The model under review builds one solid part; all positions refer to its coordinate system, in mm. A direction names the side the tool comes from. Round coordinates to 2 decimals unless told otherwise and drop trailing zeros. Write each loop counter-clockwise with the first axis right and the second up, starting at its lowest first coordinate (ties: lowest second). Pieces come first, ordered by that corner, then holes. Notation, with made-up numbers: (76, 53.5) - (125, 53.5) arc R14 ccw to (125, 73.5) - close; hole circle Ø6 at (-19, -15). An arc over 180 degrees is marked (long way). One line per question, with ' | ' between items. Start each with the question number.
```python
from build123d import *

# Parameters (mm, degrees)
SKETCH_1_W          = 23
SKETCH_1_H          = 32
EXTRUDE_1_DEPTH     = 6.5
SKETCH_3_W          = 18.5
SKETCH_3_H          = 32
CUT_EXTRUDE_1_DEPTH = 3.8
SKETCH_4_W          = 23.00306398
SKETCH_4_H          = 3
CUT_EXTRUDE_2_DEPTH = 2
SKETCH_5_R          = 0.6
CUT_EXTRUDE_3_DEPTH = 7.5
SKETCH_6_W          = 5
SKETCH_6_H          = 7
EXTRUDE_2_DEPTH     = 8.5
FILLET_1_R          = 1
SKETCH_7_R          = 0.5
CUT_EXTRUDE_4_DEPTH = 24
FILLET_2_R          = 2
FILLET_3_R          = 1
SKETCH_8_W          = 4
SKETCH_8_H          = 5
CUT_EXTRUDE_5_DEPTH = 16
SKETCH_9_R          = 1
CUT_EXTRUDE_6_DEPTH = 3
SKETCH_10_W         = 1
SKETCH_10_H         = 28
CUT_EXTRUDE_7_DEPTH = 7.5


with BuildPart() as part:
    # 草图1 → 凸台-拉伸1 (new body)
    with BuildSketch(Plane(origin=(0, 0, 0), x_dir=(1, 0, 0), z_dir=(0, 1, 0))):
        Rectangle(SKETCH_1_W, SKETCH_1_H)
    extrude(amount=EXTRUDE_1_DEPTH)

    # 草图3 → 切除-拉伸1 (cut)
    with BuildSketch(Plane.XZ):
        Rectangle(SKETCH_3_W, SKETCH_3_H)
    extrude(amount=-CUT_EXTRUDE_1_DEPTH, mode=Mode.SUBTRACT)

    # 草图4 → 切除-拉伸2 (cut)
    with BuildSketch(Plane.XZ):
        with Locations((0.00153199, 3.5)):
            Rectangle(SKETCH_4_W, SKETCH_4_H)
        with Locations((0.00153199, -3.5)):
            Rectangle(SKETCH_4_W, SKETCH_4_H)
    extrude(amount=-CUT_EXTRUDE_2_DEPTH, mode=Mode.SUBTRACT)

    # 草图5 → 切除-拉伸3 (cut, through all)
    with BuildSketch(Plane.XZ):
        with Locations((-10.375, -8)):
            Circle(SKETCH_5_R)
        with Locations((10.375, -8)):
            Circle(SKETCH_5_R)
        with Locations((10.375, 8)):
            Circle(SKETCH_5_R)
        with Locations((-10.375, 8)):
            Circle(SKETCH_5_R)
    extrude(amount=-CUT_EXTRUDE_3_DEPTH, mode=Mode.SUBTRACT)

    # 草图6 → 凸台-拉伸2 (add)
    with BuildSketch(Plane(origin=(0, 6.5, 0), x_dir=(1, 0, 0), z_dir=(0, 1, 0))):
        with Locations((9, 0)):
            Rectangle(SKETCH_6_W, SKETCH_6_H)
    extrude(amount=EXTRUDE_2_DEPTH)

    # 圆角1
    fillet_1_edges = [part.edges().sort_by_distance(p)[0] for p in [
        (10.375, 2, 5),
        (-10.375, 2, 5),
        (10.375, 2, 2),
        (-10.375, 2, 2),
        (10.375, 2, -5),
        (-10.375, 2, -5),
        (10.375, 2, -2),
        (-10.375, 2, -2),
    ]]
    fillet(fillet_1_edges, radius=FILLET_1_R)

    # 草图7 → 切除-拉伸4 (cut, through all)
    with BuildSketch(Plane(origin=(11.5, 0, 0), x_dir=(0, 0, -1), z_dir=(1, 0, 0))):
        with Locations((-2, 10.75)):
            Circle(SKETCH_7_R)
        with Locations((2, 10.75)):
            Circle(SKETCH_7_R)
    extrude(amount=-CUT_EXTRUDE_4_DEPTH, mode=Mode.SUBTRACT)

    # 圆角2
    fillet_2_edges = [part.edges().sort_by_distance(p)[0] for p in [
        (9, 15, 3.5),
        (9, 15, -3.5),
    ]]
    fillet(fillet_2_edges, radius=FILLET_2_R)

    # 圆角3
    fillet_3_edges = [part.edges().sort_by_distance(p)[0] for p in [
        (6.5, 6.5, 0),
        (9, 6.5, 3.5),
        (9, 6.5, -3.5),
    ]]
    fillet(fillet_3_edges, radius=FILLET_3_R)

    # 草图8 → 切除-拉伸5 (cut, through all)
    with BuildSketch(Plane.XZ):
        with Locations((9.5, 13.5)):
            Rectangle(SKETCH_8_W, SKETCH_8_H)
        with Locations((9.5, -13.5)):
            Rectangle(SKETCH_8_W, SKETCH_8_H)
    extrude(amount=-CUT_EXTRUDE_5_DEPTH, mode=Mode.SUBTRACT)

    # 草图9 → 切除-拉伸6 (cut)
    with BuildSketch(Plane(origin=(0, 6.5, 0), x_dir=(1, 0, 0), z_dir=(0, 1, 0))):
        with Locations((-10.375, 8)):
            Circle(SKETCH_9_R)
        with Locations((10.375, 8)):
            Circle(SKETCH_9_R)
        with Locations((-10.375, -8)):
            Circle(SKETCH_9_R)
        with Locations((10.375, -8)):
            Circle(SKETCH_9_R)
    extrude(amount=-CUT_EXTRUDE_6_DEPTH, mode=Mode.SUBTRACT)

    # 草图10 → 切除-拉伸7 (cut, through all)
    with BuildSketch(Plane(origin=(0, 6.5, 0), x_dir=(1, 0, 0), z_dir=(0, 1, 0))):
        with Locations((-8, 0)):
            Rectangle(SKETCH_10_W, SKETCH_10_H)
        with Locations((-5.5, 0)):
            Rectangle(SKETCH_10_W, SKETCH_10_H)
        with Locations((-3, 0)):
            Rectangle(SKETCH_10_W, SKETCH_10_H)
        with Locations((-0.5, 0)):
            Rectangle(SKETCH_10_W, SKETCH_10_H)
        with Locations((2, 0)):
            Rectangle(SKETCH_10_W, SKETCH_10_H)
        with Locations((4.5, 0)):
            Rectangle(SKETCH_10_W, SKETCH_10_H)
    extrude(amount=-CUT_EXTRUDE_7_DEPTH, mode=Mode.SUBTRACT)


solid = part.part
```
1. Add section B-B, the plane z = 5.5. State how many separate pieces and enclosed holes the cut face has, then the cut area to 3 significant figures.
2. Add section D-D, the plane x = 8. Write out the cut boundary in (y, z), then the cut area to 3 significant figures.
3. Wall thickness on line 1 along X through (y, z) = (2, -2); line 2 along Y through (x, z) = (-9.75, -12); line 3 along Y through (x, z) = (-2, 1.5): over which ranges is each line inside the solid? List them lowest first. Write a range as [from, to].
4. Add section C-C, the plane y = 10.75. Write out the cut boundary in (x, z).
5. Clearance check with flat-ended pins moving along their axes: P1, Ø10, axis at x = -2.5, z = -11.5, coming from the +Y side; P2, Ø0.5, axis at x = 10.5, z = 3.5, coming from the -Y side; P3, Ø12, axis at x = -8, z = 2, coming from the -Y side; P4, Ø3, axis at x = -3, z = 2, coming from the -Y side. State where each tip first meets the part, or that it passes through.
6. Machinability: for faces 1 (the face through (4, 5, 0)), 2 (the face through (-10.4, 0.5, 2)), 3 (the face through (9, 10, 3.5)), which of the approach directions +Z, -Z, +X, -X, +Y, -Y give a long, thin tool a straight path to every point of the face, cutting with its end or side? Answer none if there is none.
7. Add section A-A, the plane y = 2.75. Write out the cut boundary in (x, z) (3 decimals).
8. The part is to be moulded in two halves that separate along Z. For faces 4 (the face through (10.391, 1.699, 2.285)), 5 (the face through (-10, 0, -11)), 6 (the face through (10, 4, 11)), say which applies: pulls with the +Z half, pulls with the -Z half, needs draft (parallel to the pull), parting line crosses it, or undercut.
Geometry check:
1) separate pieces: 7 | enclosed holes: 0 | area: 63.0 mm2
2) outline: (3.8, -11) - (6.5, -11) - (6.5, -4.5) arc R1 cw to (7.5, -3.5) - (13, -3.5) arc R2 ccw to (15, -1.5) - (15, 1.5) arc R2 ccw to (13, 3.5) - (7.5, 3.5) arc R1 cw to (6.5, 4.5) - (6.5, 11) - (3.8, 11) - close; hole circle Ø1 at (10.75, -2); hole circle Ø1 at (10.75, 2) | area: 116 mm2
3) line 1: x = [-11.5, -9.25], [9.25, 11.5] | line 2: y = [0, 6.5] | line 3: y = [3.8, 6.5]
4) outline: (6.5, -3.5) - (11.5, -3.5) - (11.5, -2.5) - (6.5, -2.5) - close; (6.5, -1.5) - (11.5, -1.5) - (11.5, 1.5) - (6.5, 1.5) - close; (6.5, 2.5) - (11.5, 2.5) - (11.5, 3.5) - (6.5, 3.5) - close
5) P1: stops at y = 6.5 | P2: stops at y = 2 | P3: stops at y = 0 | P4: stops at y = 3.8
6) face 1: +Y, -Y | face 2: +X, -X, -Y | face 3: +Z, +X, -X, +Y
7) outline: (-11.5, -16) - (-9.25, -16) - (-9.25, 16) - (-11.5, 16) - close; (9.25, -11) - (11.5, -11) - (11.5, 11) - (9.25, 11) - close; hole circle Ø1.2 at (-10.375, -8); hole circle Ø1.2 at (-10.375, 8); hole circle Ø1.2 at (10.375, -8); hole circle Ø1.2 at (10.375, 8)
8) face 4: undercut | face 5: needs draft | face 6: pulls with the +Z half
